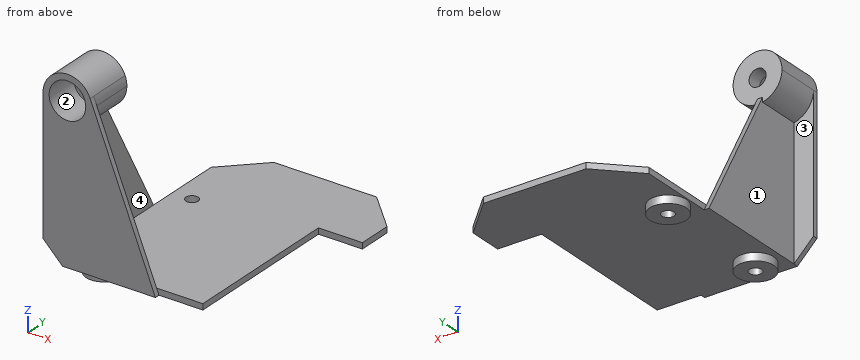
```python
from build123d import *

# Parameters (mm, degrees)
F0_R      = 1.25
F1_DEPTH  = 1.2
F2_R      = 3.75
F2_R_2    = 1.25
F3_DEPTH  = 1.6
F4_R      = 1.75
F5_DEPTH  = 1
F6_DEPTH  = 9
F8_DEPTH  = 1
F10_DEPTH = 1.001
F11_R     = 3.75
F12_DEPTH = 7
F13_W     = 9
F13_H     = 33
F14_DEPTH = 2.801


with BuildPart() as f1:
    # F0 (on Top) → F1 (new body)
    with BuildSketch(Plane.XY):
        Polygon((0, 20), (0, 0), (36, 0), (36, 48.5), (0, 48.5), align=None)
        with Locations((4, 4)):
            Circle(F0_R, mode=Mode.SUBTRACT)
        with Locations((4, 29)):
            Circle(F0_R, mode=Mode.SUBTRACT)
    extrude(amount=F1_DEPTH)

    # F2 (on face) → F3 (join)
    with BuildSketch(Plane.XY):
        with Locations((4, 29)):
            Circle(F2_R)
        with Locations((4, 29)):
            Circle(F2_R_2, mode=Mode.SUBTRACT)
        with Locations((4, 4)):
            Circle(F2_R)
        with Locations((4, 4)):
            Circle(F2_R_2, mode=Mode.SUBTRACT)
    extrude(amount=-F3_DEPTH)

    # F4 (on Front) → F5 (join)
    with BuildSketch(Plane.XZ):
        with BuildLine():
            ThreePointArc((4.641671, 33.358733), (4.909601, 32.446479), (5, 31.5))
            ThreePointArc((5, 31.5), (0, 26.5), (-5, 31.5))
            Line((-5, 31.5), (-5, 0))
            Line((-5, 0), (0, 0))
            Line((0, 0), (18, 0))
            Line((18, 0), (4.641671, 33.358733))
        make_face()
        with BuildLine():
            ThreePointArc((-5, 31.5), (0, 26.5), (5, 31.5))
            ThreePointArc((5, 31.5), (4.909601, 32.446479), (4.641671, 33.358733))
            ThreePointArc((4.641671, 33.358733), (-0.946479, 36.409601), (-5, 31.5))
        make_face()
        with Locations((0, 31.5)):
            Circle(F4_R, mode=Mode.SUBTRACT)
    extrude(amount=F5_DEPTH)

    # F4 (on Front) → F6 (join)
    with BuildSketch(Plane.XZ):
        with BuildLine():
            ThreePointArc((-5, 31.5), (0, 26.5), (5, 31.5))
            ThreePointArc((5, 31.5), (4.909601, 32.446479), (4.641671, 33.358733))
            ThreePointArc((4.641671, 33.358733), (-0.946479, 36.409601), (-5, 31.5))
        make_face()
        with Locations((0, 31.5)):
            Circle(F4_R, mode=Mode.SUBTRACT)
    extrude(amount=-F6_DEPTH)

    # F7 (on face) → F8 (join)
    with BuildSketch(Plane(origin=(0, 0, 0), x_dir=(0, -1, 0), z_dir=(-1, 0, 0))):
        Polygon((-9, 27.5), (-24.25, 0), (0, 0), (0, 27.5), align=None)
    extrude(amount=F8_DEPTH)

    # F9 (on face) → F10 (cut, through all)
    with BuildSketch(Plane.XZ):
        Polygon((-5, 0), (-1, 0), (-5, 4), align=None)
    extrude(amount=F10_DEPTH, mode=Mode.SUBTRACT)

    # F11 (on face) → F12 (cut)
    with BuildSketch(Plane.XZ.offset(1)):
        with Locations((0, 31.5)):
            Circle(F11_R)
    extrude(amount=-F12_DEPTH, mode=Mode.SUBTRACT)

    # F13 (on face) → F14 (cut, through all)
    with BuildSketch(Plane.XY.offset(1.2)):
        Polygon((36, 48.5), (0, 48.5), (0, 47.5), (0, 40.014719), (7.485281, 47.5), (28.514719, 47.5), (36, 40.014719), (36, 47.5), align=None)
        with Locations((31.5, 16.5)):
            Rectangle(F13_W, F13_H)
    extrude(amount=-F14_DEPTH, mode=Mode.SUBTRACT)


solid = f1.part
```
Verification items for the finished model (mm, model axes). Face numbers are marked on the shaded views. Coordinates: 2 decimals unless noted, no trailing zeros. Write each loop counter-clockwise with the first axis right and the second up, starting at its lowest first coordinate (ties: lowest second). Pieces come first, ordered by that corner, then holes. Notation, with made-up numbers: M 24,32 L 74,32 A6 cw 74,40 Z; hole C -33.75,64.25 d3. An arc over 180 degrees is marked long. One line per item, written item: value.
Item 1: Section check C-C, the plane x = 21. Record the boundary of the cut face in (y, z), plus the area to 3 significant figures.
Check sheet entries:
outline: M 0,0 L 47.5,0 L 47.5,1.2 L 0,1.2 Z
area: 57.0 mm^2
Item 2: Mould release check, pull along X, two halves, no side actions. Record for the marked faces 1, 2, 3 and 4: pulls with the +X half, pulls with the -X half, needs draft (parallel to the pull), parting line crosses it, or undercut.
Check sheet entries:
face 1: pulls with the -X half
face 2: undercut
face 3: needs draft
face 4: pulls with the +X half
Item 3: Scan lines: line 1 along Y through (x, z) = (4, -0.2); line 2 along Y through (x, z) = (7, 10.5); line 3 along Y through (x, z) = (4, 0.35). Record each from-to range of solid material in increasing order.
Check sheet entries:
line 1: y = 0.25 to 2.75, 5.25 to 7.75, 25.25 to 27.75, 30.25 to 32.75
line 2: y = -1 to 0
line 3: y = -1 to 2.75, 5.25 to 27.75, 30.25 to 44.01
Item 4: Section check D-D, the plane z = 18. Record the boundary of the cut face in (x, y), plus the area to 3 significant figures.
Check sheet entries:
outline: M -5,-1 L 10.79,-1 L 10.79,0 L 0,0 L 0,14.27 L -1,14.27 L -1,0 L -5,0 Z
area: 30.1 mm^2
Item 5: Gauge pin test, flat ends, axial feed: pin 1 Ø3 at (x, z) = (-3.5, 20.5) entering from +Y; pin 2 Ø1 at (y, z) = (8.5, 14.5) entering from +X; pin 3 Ø12 at (x, z) = (0, 31.5) entering from +Y. Record the tip position at first contact, or that the pin passes through.
Check sheet entries:
pin 1: stops at y = 0
pin 2: stops at x = 0
pin 3: stops at y = 10.11
Item 6: Section check A-A, the plane y = 4. Record the boundary of the cut face in (x, z), plus the area to 3 significant figures.
Check sheet entries:
outline: M -1,0 L 0.25,0 L 0.25,-1.6 L 2.75,-1.6 L 2.75,1.2 L 0,1.2 L 0,26.5 A5 ccw 5,31.5 A5 ccw 4.64,33.36 A5 ccw long -1,26.6 Z; M 5.25,-1.6 L 7.75,-1.6 L 7.75,0 L 27,0 L 27,1.2 L 5.25,1.2 Z; hole C 0,31.5 d7.5
area: 98.3 mm^2
Item 7: Section check B-B, the plane y = 29. Record the boundary of the cut face in (x, z).
Check sheet entries:
outline: M 0,0 L 0.25,0 L 0.25,-1.6 L 2.75,-1.6 L 2.75,1.2 L 0,1.2 Z; M 5.25,-1.6 L 7.75,-1.6 L 7.75,0 L 27,0 L 27,1.2 L 5.25,1.2 Z
